```python
from build123d import *

# Parameters (mm, degrees)
F0_R     = 101.6
F0_R_2   = 7.9375
F1_DEPTH = 6.35
F2_R     = 101.6
F2_R_2   = 95.25
F2_R_3   = 12.7
F2_R_4   = 7.9375
F3_DEPTH = 19.05


with BuildPart() as f1:
    # F0 (on Front) → F1 (new body)
    with BuildSketch(Plane.XZ):
        Circle(F0_R)
        Circle(F0_R_2, mode=Mode.SUBTRACT)
    extrude(amount=F1_DEPTH)

    # F2 (on face) → F3 (join)
    with BuildSketch(Plane.XZ.offset(6.35)):
        Circle(F2_R)
        Circle(F2_R_2, mode=Mode.SUBTRACT)
        Circle(F2_R_3)
        Circle(F2_R_4, mode=Mode.SUBTRACT)
    extrude(amount=F3_DEPTH)

    # F4: F1 across plane


with BuildPart() as f1_1:
    add(f1.part)
    add(f1.part.mirror(Plane.XZ))


solid = f1_1.part
```
For this review, take the finished solid that the model builds, in its own axes (mm). A direction names the side the tool comes from. Coordinates: 2 decimals unless noted, no trailing zeros. Order: outer loops, then holes, each group sorted by start corner. A loop starts at its lowest first (then second) coordinate and runs counter-clockwise, first axis right, second up. Notation, with made-up numbers: (-22.75, 53.25) - (15.25, 53.25) arc R18 ccw to (15.25, 80.25) - close; hole circle Ø10 at (-8.75, 55.5). An arc over 180 degrees is marked (long way). Answer as a JSON object with one key per item and string values. Group by question number.
1. Clearance check with flat-ended pins moving along their axes: P1, Ø3, axis at x = 16.5, z = 38.5, coming from the +Y side; P2, Ø3, axis at y = 14, z = 10, coming from the +X side; P3, Ø1, axis at x = 56.5, y = 18.5, coming from the +Z side. State where each tip first meets the part, or that it passes through.
2. The part is to be moulded in two halves that separate along Z. For faces 4 (the cylindrical face through (-22.025, -0.356, -99.184)), 5 (the flat face through (-91, 25.4, -30)), 6 (the flat face through (20, 6.35, 1)), 7 (the cylindrical face through (-2.75, -15.74, -12.4)), say which applies: pulls with the +Z half, pulls with the -Z half, needs draft (parallel to the pull), parting line crosses it, or undercut.
3. For faces 1 (the flat face through (-91, -25.4, -30)), 2 (the cylindrical face through (-75.587, -15.742, -57.958)), 3 (the cylindrical face through (-75.587, 15.742, -57.958)), list the 3-axis set-ups (+Z, -Z, +X, -X, +Y, -Y) from which the entire face can be reached by the end or side of a thin tool; tool diameter is ignored.
4. We need section D-D on x = 59. State the section outline as (y, z) points.
5. We need section B-B on x = 0. State the section outline as (y, z) points, then the cut area to 3 significant figures.
6. For probe 1 along Z at (x, y) = (0, -16); probe 2 along Z at (x, y) = (-3, 10.5); probe 3 along Y at (x, z) = (20.5, -72), list the stretches that pass through material, from the lowest coordinate up.
7. We need section C-C on y = 2. State the section outline as (x, z) points (1 decimal), then the cut area to 3 significant figures.
8. We need section A-A on z = 0. State the section outline as (x, y) points.
Final values:
{
 "1": {"P1": "y = 6.35", "P2": "x = 101.24", "P3": "z = 84.77"},
 "2": {"face 4": "parting line crosses it", "face 5": "needs draft", "face 6": "undercut", "face 7": "undercut"},
 "3": {"face 1": "+Z, -Z, +X, -X, -Y", "face 2": "-Y", "face 3": "+Y"},
 "4": {"outline": "(-25.4, -82.71) - (25.4, -82.71) - (25.4, -74.78) - (6.35, -74.78) - (6.35, 74.78) - (25.4, 74.78) - (25.4, 82.71) - (-25.4, 82.71) - (-25.4, 74.78) - (-6.35, 74.78) - (-6.35, -74.78) - (-25.4, -74.78) - close"},
 "5": {"outline": "(-25.4, -101.6) - (25.4, -101.6) - (25.4, -95.25) - (6.35, -95.25) - (6.35, -12.7) - (25.4, -12.7) - (25.4, -7.94) - (-25.4, -7.94) - (-25.4, -12.7) - (-6.35, -12.7) - (-6.35, -95.25) - (-25.4, -95.25) - close; (-25.4, 7.94) - (25.4, 7.94) - (25.4, 12.7) - (6.35, 12.7) - (6.35, 95.25) - (25.4, 95.25) - (25.4, 101.6) - (-25.4, 101.6) - (-25.4, 95.25) - (-6.35, 95.25) - (-6.35, 12.7) - (-25.4, 12.7) - close", "area": "3,230 mm²"},
 "6": {"probe 1": "-101.6 to -95.25, -12.7 to -7.94, 7.94 to 12.7, 95.25 to 101.6", "probe 2": "-101.56 to -95.2, -12.34 to -7.35, 7.35 to 12.34, 95.2 to 101.56", "probe 3": "-6.35 to 6.35"},
 "7": {"outline": "circle Ø203.2 at (0, 0); hole circle Ø15.9 at (0, 0)", "area": "32,200 mm²"},
 "8": {"outline": "(-101.6, -25.4) - (-95.25, -25.4) - (-95.25, -6.35) - (-12.7, -6.35) - (-12.7, -25.4) - (-7.94, -25.4) - (-7.94, 25.4) - (-12.7, 25.4) - (-12.7, 6.35) - (-95.25, 6.35) - (-95.25, 25.4) - (-101.6, 25.4) - close; (7.94, -25.4) - (12.7, -25.4) - (12.7, -6.35) - (95.25, -6.35) - (95.25, -25.4) - (101.6, -25.4) - (101.6, 25.4) - (95.25, 25.4) - (95.25, 6.35) - (12.7, 6.35) - (12.7, 25.4) - (7.94, 25.4) - close"}
}
